Read the model definition and answer for the solid it produces. Units are mm, in the model's axes. Face numbers are marked on the shaded views. A direction names the side the tool comes from. Round coordinates to 2 decimals unless told otherwise and drop trailing zeros. Loops run counter-clockwise (first coordinate to the right, second up) from the corner with the lowest first, then second, coordinate; pieces in that order, holes last. Notation, with made-up numbers: (5.5, 39.25) - (41.5, 39.25) arc R28 ccw to (41.5, 68.25) - close; hole circle Ø11 at (10, 0.5). An arc over 180 degrees is marked (long way). Answer as CSV lines item,"result".
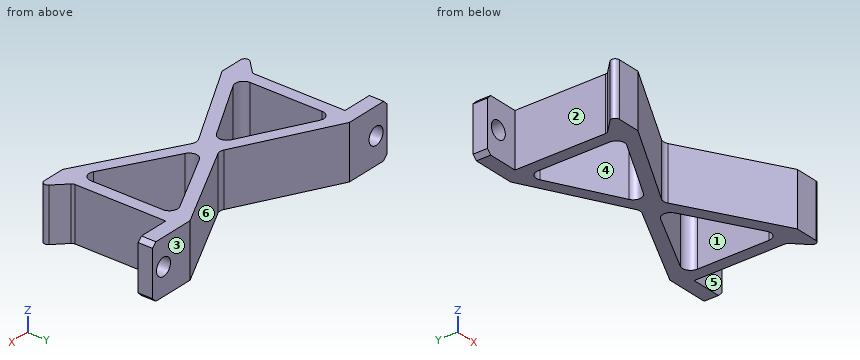
Autodesk Inventor part; units mm, degrees
ref_plane "YZ Plane" through (0, 0, 0) normal (1, 0, 0) x (0, 1, 0)
ref_plane "XZ Plane" through (0, 0, 0) normal (0, 1, 0) x (-1, 0, 0)
ref_plane "XY Plane" through (0, 0, 0) normal (0, 0, 1) x (1, 0, 0)
sketch "Sketch1" plane through (0, 0, 0) normal (0, 0, 1) x (1, 0, 0)
  line L0 (-35.3, 0) -> (-27, 0)
  line L1 (-27, 0) -> (-27, -3.5)
  line L2 (-27, -3.5) -> (-35.3, -3.5)
  line L3 (-35.3, -3.5) -> (-35.3, 0)
  line L4 (-27, 0) -> (-24, 0)
  line L5 (-24, 0) -> (-24, -31)
  line L6 (-24, -31) -> (-27, -31)
  line L7 (-27, -31) -> (-27, 0)
  line L8 (-27, -31) -> (-32, -31)
  line L9 (-32, -31) -> (-27, -26)
  line L10 (-24, -31) -> (36.4267, -31) construction
  line L11 (0, 0) -> (0, -31)
  line L12 (-24, 0) -> (31.066, 0) construction
  line L13 (-24, -31) -> (0, -17.6011)
  line L14 (-24, -27.5641) -> (-1.4552, -14.9777)
  line L15 (-24, 0) -> (0, -12.3526)
  line L16 (-1.4552, -14.9777) -> (-24, -3.374)
  line L17 (35.3, 0) -> (27, 0)
  line L18 (27, 0) -> (27, -3.5)
  line L19 (27, -3.5) -> (35.3, -3.5)
  line L20 (35.3, -3.5) -> (35.3, 0)
  line L21 (27, 0) -> (24, 0)
  line L22 (24, 0) -> (24, -31)
  line L23 (24, -31) -> (27, -31)
  line L24 (27, -31) -> (27, 0)
  line L25 (27, -31) -> (32, -31)
  line L26 (32, -31) -> (27, -26)
  line L27 (24, -31) -> (0, -17.6011)
  line L28 (24, -27.5641) -> (1.4552, -14.9777)
  line L29 (24, 0) -> (0, -12.3526)
  line L30 (1.4552, -14.9777) -> (24, -3.374)
  dimension "d0" = 8.3
  dimension "d1" = 3.5
  dimension "d2" = 27
  dimension "d3" = 3
  dimension "d4" = 31
  dimension "d5" = 5
  dimension "d7" = 45
  dimension "d13" = 0
  dimension "d17" = 3
  dimension "d18" = 3
extrude "Extrusion1" add sketch "Sketch1" along normal blind 13 contours L0 L1 L2 L3 | L4 L5 L6 L7 L1 | L15 L11 L13 L5 L14 L16 | L7 L8 L9 | L29 L22 L30 L28 L27 L11 | L21 L18 L24 L23 L22 | L17 L20 L19 L18 | L24 L26 L25
sketch "Sketch2" plane through (-35.3, 0, 0) normal (0, 1, 0) x (1, 0, 0)
  line L0 (0, 0) -> (11.3, 0)
  line L1 (0, 0) -> (0, -13)
  line L2 (11.3, -13) -> (0, -13)
  line L3 (11.3, 0) -> (11.3, -13)
  line L4 (59.3, 0) -> (70.6, 0)
  line L5 (59.3, 0) -> (59.3, -13)
  line L6 (70.6, -13) -> (59.3, -13)
  line L7 (70.6, 0) -> (70.6, -13)
  point P0 (35.3, 0)
  point P1 (3.3, -6.5)
  point P2 (67.3, -6.5)
  dimension "d21" = 64
  dimension "d22" = 70.6
  dimension "d23" = 3.3
  dimension "d24" = 6.5
  dimension "d25" = 13
hole "Hole1" at (-32, 0, 6.5) at (32, 0, 6.5) direction (0, -1, 0) diameter 4.2 depth 15 tip angle 118
fillet "Fillet1" radius 2 8 edges at (0, -12.3526, 6.5) (0, -17.6011, 6.5) (1.4552, -14.9777, 6.5) (-1.4552, -14.9777, 6.5) (-24, -27.5641, 6.5) (-24, -3.374, 6.5) (24, -3.374, 6.5) (24, -27.5641, 6.5)
fillet "Fillet1" radius 1 4 edges at (-27, -26, 6.5) (-32, -31, 6.5) (27, -26, 6.5) (32, -31, 6.5)
chamfer "Chamfer1" distance 1 angle 45 4 edges at (35.3, -1.75, 13) (35.3, -1.75, 0) (-35.3, -1.75, 0) (-35.3, -1.75, 13)
equation "\"d16\" = d12"
properties part number "3DP_PLA_Turbine_stand"
1) Each of these flat-tipped pins is pushed along its axis until it touches: P1, Ø4, axis at y = -11.5, z = 6, coming from the -X side; P2, Ø1.5, axis at x = -13, y = -18.5, coming from the -Z side; P3, Ø2.5, axis at x = -32.5, z = 5.5, coming from the -Y side; P4, Ø4, axis at x = -32, z = 6.5, coming from the -Y side. Where does it stop, or does it pass through?
Entries:
P1,"stops at x = -27"
P2,"passes through"
P3,"stops at y = -3.5"
P4,"stops at y = -30.91"
2) Find the intervals of material crossed by line 1 (X direction, y = -2.3, z = 6.5); line 2 (X direction, y = -24.5, z = 10); line 3 (Z direction, x = 32, y = -1.35), in increasing order.
Entries:
line 1,"x = -35.3 to -34.1, -29.9 to -19.53, 19.53 to 29.9, 34.1 to 35.3"
line 2,"x = -27 to -23.97, -18.51 to -12.36, 12.36 to 18.51, 23.97 to 27"
line 3,"z = 0 to 4.4, 8.6 to 13"
3) A cutting plane is placed at B-B, the plane y = -21.5. Determine the outline of the cut face in (x, z).
Entries:
outline,"(-27, 0) - (-24, 0) - (-24, 13) - (-27, 13) - close; (-13.14, 0) - (-6.98, 0) - (-6.98, 13) - (-13.14, 13) - close; (6.98, 0) - (13.14, 0) - (13.14, 13) - (6.98, 13) - close; (24, 0) - (27, 0) - (27, 13) - (24, 13) - close"
4) A cutting plane is placed at A-A, the plane x = -32. Determine the outline of the cut face in (y, z).
Entries:
outline,"(-3.5, 0) - (0, 0) - (0, 4.4) - (-3.5, 4.4) - close; (-3.5, 8.6) - (0, 8.6) - (0, 13) - (-3.5, 13) - close"
5) A cutting plane is placed at C-C, the plane z = 6.5. Count the separate pieces of the cut face and the enclosed holes in it, plus the area to 3 significant figures.
Entries:
separate pieces,"3"
enclosed holes,"2"
area,"579 mm^2"
6) A tool of negligible diameter and unlimited length cuts with its end or side. For the marked faces 4, 5 and 6, from which of +Z, -Z, +X, -X, +Y, -Y can it reach the whole face along a straight path? Write none if from no direction.
Entries:
face 4,"+Z, -Z"
face 5,"+Z, -Z, +X"
face 6,"+Z, -Z, +Y"
7) A cutting plane is placed at D-D, the plane y = -14. Determine the outline of the cut face in (x, z), plus the area to 3 significant figures.
Entries:
outline,"(-27, 0) - (-24, 0) - (-24, 13) - (-27, 13) - close; (-3.98, 0) - (3.98, 0) - (3.98, 13) - (-3.98, 13) - close; (24, 0) - (27, 0) - (27, 13) - (24, 13) - close"
area,"182 mm^2"
8) The mould has two halves that part along X. Classify the marked faces 1, 2 and 3: pulls with the +X half, pulls with the -X half, needs draft (parallel to the pull), parting line crosses it, or undercut.
Entries:
face 1,"undercut"
face 2,"pulls with the -X half"
face 3,"needs draft"
